Model file for the job. Use its own axes, mm. A direction names the side the tool comes from. Coordinates: 2 decimals unless noted, no trailing zeros. Loops run counter-clockwise (first coordinate to the right, second up) from the corner with the lowest first, then second, coordinate; pieces in that order, holes last.
from build123d import *

# Parameters (mm, degrees)
F0_W        = 28
F0_H        = 20
F1_DEPTH    = 68
F3_DEPTH    = 15
F2_W        = 24
F2_H        = 100
F4_DEPTH    = 18
F5_T1_DEPTH = 166
F6_R        = 1.6
F7_DEPTH    = 140
F6_R_2      = 2.75
F8_DEPTH    = 3
F9_R        = 2.75
F9_R_2      = 1.6
F10_DEPTH   = 3


# Not quite as in the source:
# - a fillet or chamfer that OpenCascade refuses, or shapes differently, is made with other operations: its cross-section is extruded or revolved along the edge and cut away or added


with BuildPart() as f1:
    # F0 (on Front) → F1 (new body, symmetric)
    with BuildSketch(Plane.XZ):
        Rectangle(F0_W, F0_H)
    extrude(amount=F1_DEPTH, both=True)

    # F2 (on face) → F3 (cut)
    with BuildSketch(Plane(origin=(0, 0, -10), x_dir=(1, 0, 0), z_dir=(0, 0, -1))):
        Polygon((12, 62), (-12, 62), (-12, 53.5), (-10.3, 53.5), (-10.3, 60.3), (10.3, 60.3), (10.3, 53.5), (12, 53.5), align=None)
        Polygon((-12, -53.5), (-12, -62), (12, -62), (12, -53.5), (10.3, -53.5), (10.3, -60.3), (-10.3, -60.3), (-10.3, -53.5), align=None)
    extrude(amount=-F3_DEPTH, mode=Mode.SUBTRACT)

    # F2 (on face) → F4 (cut)
    with BuildSketch(Plane(origin=(0, 0, -10), x_dir=(1, 0, 0), z_dir=(0, 0, -1))):
        Rectangle(F2_W, F2_H)
    extrude(amount=-F4_DEPTH, mode=Mode.SUBTRACT)

    # F5: fillet of radius 6 on 4 edges, made by hand

    # F5_s2 → F5_t1 (cut)
    with BuildSketch(Plane.XZ.offset(-83)):
        with BuildLine():
            ThreePointArc((-8, 10), (-12.2426406871, 8.2426406871), (-14, 4))
            Line((-14, 4), (-14, 10))
            Line((-14, 10), (-8, 10))
        make_face()
        with BuildLine():
            ThreePointArc((8, 10), (12.2426406871, 8.2426406871), (14, 4))
            Line((14, 4), (14, 10))
            Line((14, 10), (8, 10))
        make_face()
        with BuildLine():
            ThreePointArc((14, -4), (12.2426406871, -8.2426406871), (8, -10))
            Line((8, -10), (14, -10))
            Line((14, -10), (14, -4))
        make_face()
        with BuildLine():
            ThreePointArc((-14, -4), (-12.2426406871, -8.2426406871), (-8, -10))
            Line((-8, -10), (-14, -10))
            Line((-14, -10), (-14, -4))
        make_face()
    extrude(amount=F5_T1_DEPTH, mode=Mode.SUBTRACT)

    # F6 (on face) → F7 (cut)
    with BuildSketch(Plane(origin=(0, 68, 0), x_dir=(-1, 0, 0), z_dir=(0, 1, 0))):
        with Locations((0, 3.4)):
            Circle(F6_R)
    extrude(amount=-F7_DEPTH, mode=Mode.SUBTRACT)

    # F6 (on face) → F8 (cut)
    with BuildSketch(Plane(origin=(0, 68, 0), x_dir=(-1, 0, 0), z_dir=(0, 1, 0))):
        with Locations((0, 3.4)):
            Circle(F6_R_2)
        with Locations((0, 3.4)):
            Circle(F6_R, mode=Mode.SUBTRACT)
    extrude(amount=-F8_DEPTH, mode=Mode.SUBTRACT)

    # F9 (on face) → F10 (cut)
    with BuildSketch(Plane.XZ.offset(68)):
        with Locations((0, 3.4)):
            Circle(F9_R)
        with Locations((0, 3.4)):
            Circle(F9_R_2, mode=Mode.SUBTRACT)
    extrude(amount=-F10_DEPTH, mode=Mode.SUBTRACT)


solid = f1.part
Q1. Slice it at A-A (y = -46). List the corners of the cut face in (x, z), and give its area (3 significant figures).
Answers:
outline: (-14, -4) arc R6 ccw to (-12, -8.47) - (-12, 8) - (12, 8) - (12, -8.47) arc R6 ccw to (14, -4) - (14, 4) arc R6 ccw to (8, 10) - (-8, 10) arc R6 ccw to (-14, 4) - close
area: 101 mm2
Q2. Slice it at C-C (x = 6). List the corners of the cut face in (y, z).
Answers:
outline: (-68, -10) - (-62, -10) - (-62, 5) - (-60.3, 5) - (-60.3, -10) - (-50, -10) - (-50, 8) - (50, 8) - (50, -10) - (60.3, -10) - (60.3, 5) - (62, 5) - (62, -10) - (68, -10) - (68, 10) - (-68, 10) - close
Q3. Mould opens along Z. For faces 3 (the cylindrical face through (0.35, -55.08, 1.84)), 4 (the flat face through (12, 1, 0)), 5 (the flat face through (0, -1, 10)), 6 (the cylindrical face through (0.35, 55.22, 1.84)) say: +Z half, -Z half, draft (parallel to the pull), parting line (faces both ways), or undercut.
Answers:
face 3: undercut
face 4: draft
face 5: +Z half
face 6: undercut
Q4. Drill centre lines: line 1 (Y direction, x = 11.75, z = -5); line 2 (Y direction, x = -3, z = -3.5); line 3 (X direction, y = 28, z = -4.5). Where is each one in solid material? Low to high.
Answers:
line 1: y = -68 to -62, -53.5 to -50, 50 to 53.5, 62 to 68
line 2: y = -68 to -62, -60.3 to -50, 50 to 60.3, 62 to 68
line 3: x = -13.98 to -12, 12 to 13.98
Q5. Which spindle directions (+Z, -Z, +X, -X, +Y, -Y) get a long thin tool onto all of the face, cutting with end or side? Do faces 1 (the flat face through (10.3, -57, -2)), 2 (the flat face through (0, 55, -10)). Say none if no direction does.
Answers:
face 1: -Z
face 2: -Z, +X, -X, +Y, -Y
Q6. Slice it at B-B (z = -2.5). List the corners of the cut face in (x, y).
Answers:
outline: (-14, -68) - (14, -68) - (14, 68) - (-14, 68) - close; hole (-12, -62) - (12, -62) - (12, -53.5) - (10.3, -53.5) - (10.3, -60.3) - (-10.3, -60.3) - (-10.3, -53.5) - (-12, -53.5) - close; hole (-12, -50) - (12, -50) - (12, 50) - (-12, 50) - close; hole (-12, 53.5) - (-10.3, 53.5) - (-10.3, 60.3) - (10.3, 60.3) - (10.3, 53.5) - (12, 53.5) - (12, 62) - (-12, 62) - close
Q7. Flat gauge pins, fed straight in: P1, Ø8, axis at x = 7.5, y = -26, coming from the -Z side; P2, Ø3.5, axis at x = 0, z = 3.4, coming from the +Y side. Where does each tip first touch, or does it go through?
Answers:
P1: stops at z = 8
P2: stops at y = 65
